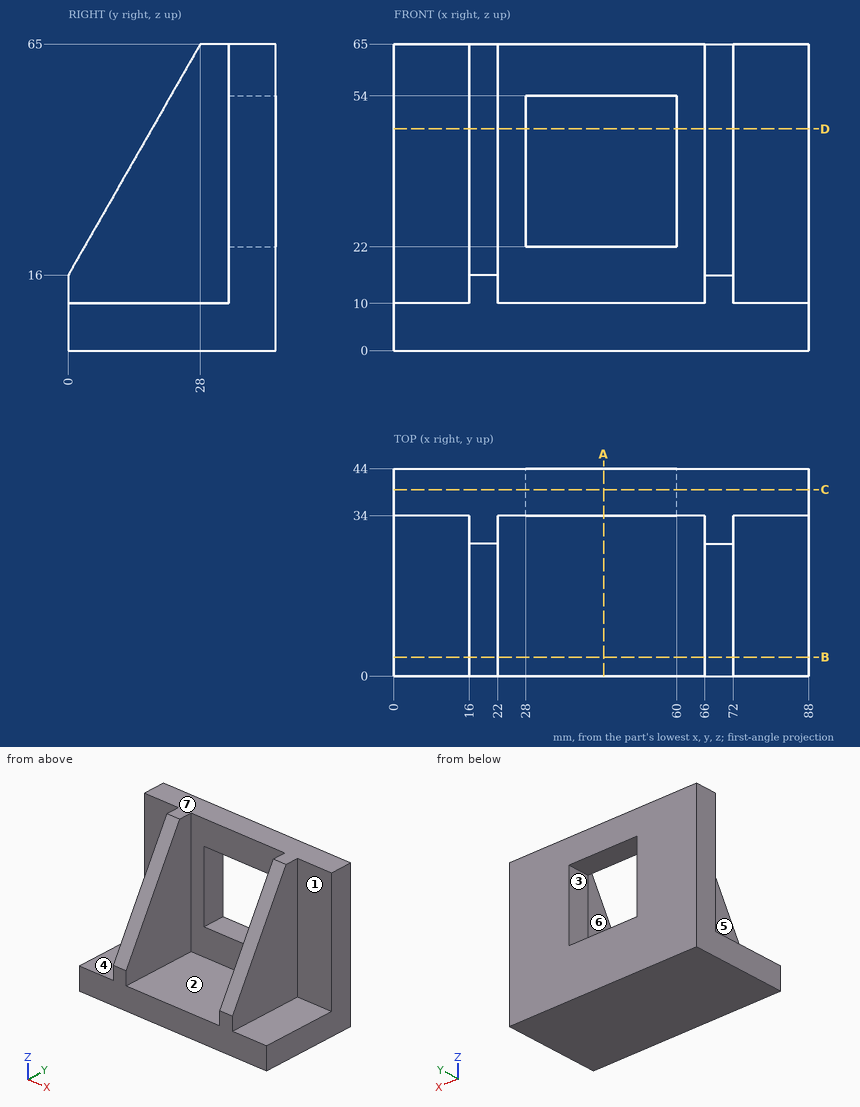
The drawing under review shows one solid part. Ordinate dimensions are in mm from its lowest x, y, z. A direction names the side the tool comes from. Give positions to 0.01 mm unless a question says otherwise; leave off trailing zeros. Order: outer loops, then holes, each group sorted by start corner. A loop starts at its lowest first (then second) coordinate and runs counter-clockwise, first axis right, second up. Notation, with made-up numbers: M -34,77 L -22,77 A31 ccw -22,107 Z; hole C -22,42.5 d3. An arc over 180 degrees is marked long. Answer in a Markdown table with one row per item. Add a question column.
1. Add section B-B on y = 4. State the section outline as (x, z) points.
2. For pin 1 Ø8 at (x, y) = (79.5, 15) entering from +Z; pin 2 Ø13 at (x, z) = (6.5, 46) entering from -Y; pin 3 Ø12 at (y, z) = (26.5, 23) entering from -X, all flat-tipped, find the tip position at first contact; note any pin that passes through.
3. To check wall thickness, follow line 1 along X through (y, z) = (33.5, 36.5); line 2 along Z through (x, y) = (36, 39.5); line 3 along X through (y, z) = (42, 48). State the ranges of each line that lie inside material, in increasing order.
4. Add section C-C on y = 39.5. State the section outline as (x, z) points, plus the area to 3 significant figures.
5. Machinability: for the marked faces 1, 2, 3 and 4, which of the approach directions +Z, -Z, +X, -X, +Y, -Y give a long, thin tool a straight path to every point of the face, cutting with its end or side? Answer none if there is none.
6. Mouldability with a two-part tool opening along X and no side actions: class the marked faces 5, 6 and 7 as released by +X, released by -X, zero draft, split by the parting line, or undercut.
7. Add section A-A on x = 44.5. State the section outline as (y, z) points.
8. Add section D-D on z = 47. State the section outline as (x, y) points.
The answers:
| question | item | result |
|---|---|---|
| 1 | outline | M 0,0 L 88,0 L 88,10 L 72,10 L 72,23 L 66,23 L 66,10 L 22,10 L 22,23 L 16,23 L 16,10 L 0,10 Z |
| 2 | pin 1 | z = 10 |
| 2 | pin 2 | y = 34 |
| 2 | pin 3 | x = 16 |
| 3 | line 1 | 16 to 22, 66 to 72 |
| 3 | line 2 | 0 to 22, 54 to 65 |
| 3 | line 3 | 0 to 28, 60 to 88 |
| 4 | outline | M 0,0 L 88,0 L 88,65 L 0,65 Z; hole M 28,22 L 60,22 L 60,54 L 28,54 Z |
| 4 | area | 4,700 mm2 |
| 5 | face 1 | +Z, +X, -Y |
| 5 | face 2 | +Z, -Y |
| 5 | face 3 | +Y, -Y |
| 5 | face 4 | +Z, -X, -Y |
| 6 | face 5 | released by -X |
| 6 | face 6 | undercut |
| 6 | face 7 | zero draft |
| 7 | outline | M 0,0 L 44,0 L 44,22 L 34,22 L 34,10 L 0,10 Z; M 34,54 L 44,54 L 44,65 L 34,65 Z |
| 8 | outline | M 0,34 L 16,34 L 16,17.71 L 22,17.71 L 22,34 L 28,34 L 28,44 L 0,44 Z; M 60,34 L 66,34 L 66,17.71 L 72,17.71 L 72,34 L 88,34 L 88,44 L 60,44 Z |
